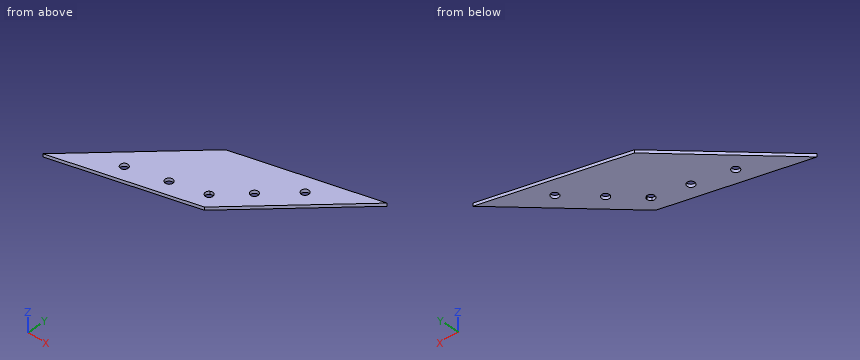
from build123d import *

# Parameters (mm, degrees)
BOSS_EXTRUDE2_DEPTH = 2
SKETCH7_R           = 2.5
CUT_EXTRUDE6_DEPTH  = 2
SKETCH8_R           = 2.5
CUT_EXTRUDE7_DEPTH  = 2
SKETCH9_R           = 2.5
CUT_EXTRUDE8_DEPTH  = 2
SKETCH10_R          = 2.5
CUT_EXTRUDE9_DEPTH  = 2
CUT_EXTRUDE10_DEPTH = 2


with BuildPart() as part:
    # Sketch1 → Boss-Extrude2 (new body)
    with BuildSketch(Plane.XY):
        Polygon((0, 0), (63.639610307, 63.639610307), (150.572934673, 86.933324366), (86.933324366, 23.293714059), align=None)
    extrude(amount=BOSS_EXTRUDE2_DEPTH)

    # Sketch7 → Cut-Extrude6 (cut)
    with BuildSketch(Plane.XY.offset(2)):
        with Locations((115.217595613, 65.72012093)):
            Circle(SKETCH7_R)
    extrude(amount=-CUT_EXTRUDE6_DEPTH, mode=Mode.SUBTRACT)

    # Sketch8 → Cut-Extrude7 (cut)
    with BuildSketch(Plane.XY.offset(2)):
        with Locations((97.539926084, 48.042451401)):
            Circle(SKETCH8_R)
    extrude(amount=-CUT_EXTRUDE7_DEPTH, mode=Mode.SUBTRACT)

    # Sketch9 → Cut-Extrude8 (cut)
    with BuildSketch(Plane.XY.offset(2)):
        with Locations((60.196988258, 26.482496195)):
            Circle(SKETCH9_R)
    extrude(amount=-CUT_EXTRUDE8_DEPTH, mode=Mode.SUBTRACT)

    # Sketch10 → Cut-Extrude9 (cut)
    with BuildSketch(Plane.XY.offset(2)):
        with Locations((36.048842601, 20.012020067)):
            Circle(SKETCH10_R)
    extrude(amount=-CUT_EXTRUDE9_DEPTH, mode=Mode.SUBTRACT)

    # Sketch11 → Cut-Extrude10 (cut)
    with BuildSketch(Plane.XY.offset(2)):
        with BuildLine():
            Line((81.756943464, 32.259468781), (80.506943464, 34.42453229))
            ThreePointArc((80.506943464, 34.42453229), (79.591879955, 31.009468781), (83.006943464, 30.094405271))
            Line((83.006943464, 30.094405271), (81.756943464, 32.259468781))
        make_face()
        with BuildLine():
            ThreePointArc((84.256943464, 32.259468781), (84.066642295, 33.216177362), (83.524710417, 34.027235734))
            Line((83.524710417, 34.027235734), (81.756943464, 32.259468781))
            Line((81.756943464, 32.259468781), (83.006943464, 30.094405271))
            ThreePointArc((83.006943464, 30.094405271), (83.922006973, 31.009468781), (84.256943464, 32.259468781))
        make_face()
        with BuildLine():
            Line((81.756943464, 32.259468781), (83.524710417, 34.027235734))
            ThreePointArc((83.524710417, 34.027235734), (82.083258945, 34.738080934), (80.506943464, 34.42453229))
            Line((80.506943464, 34.42453229), (81.756943464, 32.259468781))
        make_face()
    extrude(amount=-CUT_EXTRUDE10_DEPTH, mode=Mode.SUBTRACT)


solid = part.part
Verification items for the finished model (mm, model axes). Round coordinates to 2 decimals unless told otherwise and drop trailing zeros. Order: outer loops, then holes, each group sorted by start corner. A loop starts at its lowest first (then second) coordinate and runs counter-clockwise, first axis right, second up. Notation, with made-up numbers: (-27.5, 10.25) -> (21.5, 10.25) arc R13 ccw to (21.5, 22.25) -> close; hole circle Ø3 at (54, 76.25). An arc over 180 degrees is marked (long way). Put each result on its own line as item: value.
1) Section check B-B (x = 129). Record the cut outline in (y, z).
Final values:
outline: (65.36, 0) -> (81.15, 0) -> (81.15, 2) -> (65.36, 2) -> close
2) Material ranges on line 1 (Y direction, x = 63, z = 0.9); line 2 (Y direction, x = 60, z = 0.7); line 3 (Y direction, x = 26, z = 0.6), recorded low to high.
Final values:
line 1: y = 16.88 to 63
line 2: y = 16.08 to 23.99, 28.97 to 60
line 3: y = 6.97 to 26
3) Section check A-A (z = 1.3). Record the cut outline in (x, y).
Final values:
outline: (0, 0) -> (86.93, 23.29) -> (150.57, 86.93) -> (63.64, 63.64) -> close; hole circle Ø5 at (36.05, 20.01); hole circle Ø5 at (60.2, 26.48); hole circle Ø5 at (81.76, 32.26); hole circle Ø5 at (97.54, 48.04); hole circle Ø5 at (115.22, 65.72)
4) Section check C-C (y = 53.5). Record the cut outline in (x, z), then the cut area to 3 significant figures.
Final values:
outline: (53.5, 0) -> (117.14, 0) -> (117.14, 2) -> (53.5, 2) -> close
area: 127 mm^2
